For this review, use the dimensioned drawing (mm, ordinates from the lowest corner) and the shaded views. A direction names the side the tool comes from. Round coordinates to 2 decimals unless told otherwise and drop trailing zeros. Write each loop counter-clockwise with the first axis right and the second up, starting at its lowest first coordinate (ties: lowest second). Pieces come first, ordered by that corner, then holes. Notation, with made-up numbers: M 17,71.5 L 58,71.5 A19 ccw 58,99.5 Z; hole C -38.75,13 d8. An arc over 180 degrees is marked long. Use CSV: the item, a comma, the result in double quotes.
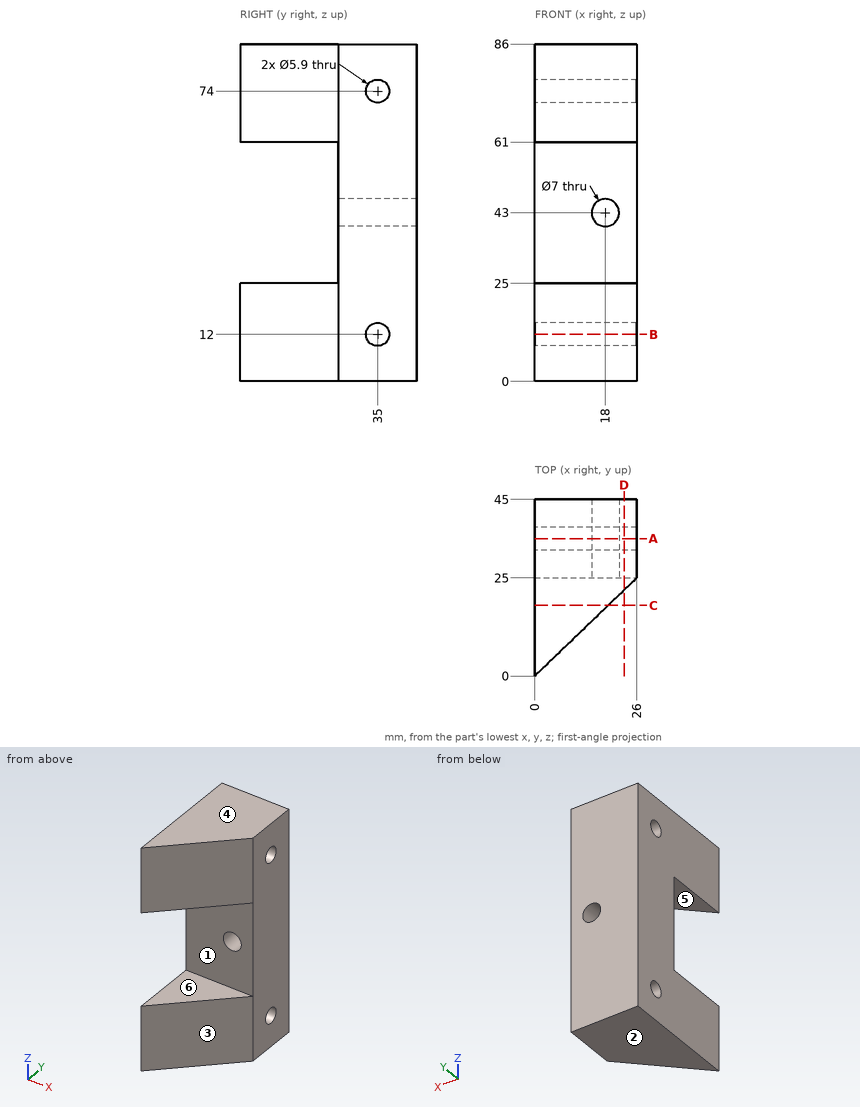
1) The part is to be moulded in two halves that separate along Z. For the marked faces 3, 4, 5 and 6, say which applies: released by +Z, released by -Z, zero draft, split by the parting line, or undercut.
Answers:
face 3,"zero draft"
face 4,"released by +Z"
face 5,"undercut"
face 6,"undercut"
2) Add section C-C on y = 18. Write out the cut boundary in (x, z).
Answers:
outline,"M 0,0 L 18.72,0 L 18.72,25 L 0,25 Z; M 0,61 L 18.72,61 L 18.72,86 L 0,86 Z"
3) Add section A-A on y = 35. Write out the cut boundary in (x, z), then the cut area to 3 significant figures.
Answers:
outline,"M 0,0 L 26,0 L 26,9.05 L 0,9.05 Z; M 0,14.95 L 26,14.95 L 26,71.05 L 0,71.05 Z; M 0,76.95 L 26,76.95 L 26,86 L 0,86 Z; hole C 18,43 d7"
area,"1,890 mm²"
4) Add section D-D on x = 22.75. Write out the cut boundary in (y, z) (3 decimals).
Answers:
outline,"M 21.875,0 L 45,0 L 45,86 L 21.875,86 L 21.875,61 L 25,61 L 25,25 L 21.875,25 Z; hole C 35,12 d5.9; hole C 35,74 d5.9"
5) Machinability: for the marked faces 1 and 2, which of the approach directions +Z, -Z, +X, -X, +Y, -Y give a long, thin tool a straight path to every point of the face, cutting with its end or side? Answer none if there is none.
Answers:
face 1,"+X, -X, -Y"
face 2,"-Z, +X, -X, +Y, -Y"
6) Add section B-B on z = 12. Write out the cut boundary in (x, y), then the cut area to 3 significant figures.
Answers:
outline,"M 0,0 L 26,25 L 26,32.05 L 0,32.05 Z; M 0,37.95 L 26,37.95 L 26,45 L 0,45 Z"
area,"692 mm²"
7) Wall thickness on line 1 along X through (y, z) = (33.5, 43); line 2 along Z through (x, y) = (9, 17); line 3 along Y through (x, z) = (12.5, 49.5): over which ranges is each line inside the solid? List them lowest first. Write a range as [from, to].
Answers:
line 1,"[0, 14.5], [21.5, 26]"
line 2,"[0, 25], [61, 86]"
line 3,"[25, 45]"
8) For pin 1 Ø10 at (y, z) = (15.5, 41.5) entering from -X; pin 2 Ø8 at (x, z) = (18, 43) entering from -Y, all flat-tipped, find the tip position at first contact; note any pin that passes through.
Answers:
pin 1,"through"
pin 2,"y = 25"
